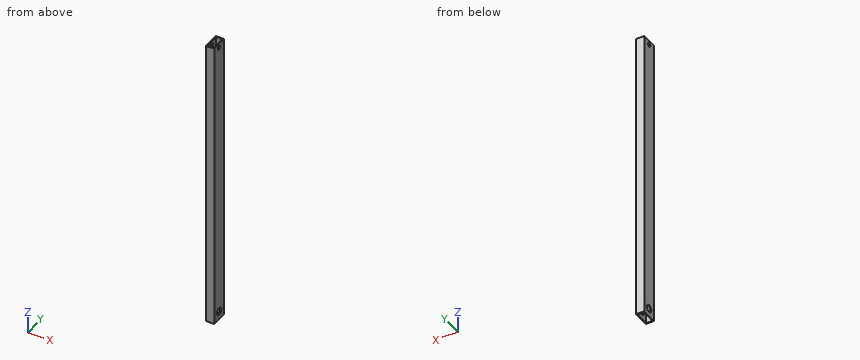
Autodesk Inventor part; units mm, degrees
ref_plane "YZ Plane" through (0, 0, 0) normal (1, 0, 0) x (0, 1, 0)
ref_plane "XZ Plane" through (0, 0, 0) normal (0, 1, 0) x (-1, 0, 0)
ref_plane "XY Plane" through (0, 0, 0) normal (0, 0, 1) x (1, 0, 0)
sketch "Sketch1" plane through (0, 0, 0) normal (0, 0, 1) x (1, 0, 0)
  line L0 (0, 0) -> (25.4, 0)
  line L1 (25.4, 0) -> (25.4, 50.8)
  line L2 (25.4, 50.8) -> (0, 50.8)
  line L3 (0, 50.8) -> (0, 0)
  dimension "d0" = 25.4
  dimension "d1" = 50.8
extrude "Extrusion1" add sketch "Sketch1" along normal blind 914.4
shell "Shell1" thickness 3.175 removed faces 2 at (8.4667, 16.9333, 0) at (8.4667, 16.9333, 914.4)
sketch "Sketch2" plane through (25.4, 0, 0) normal (1, 0, 0) x (0, 0, -1)
  circle A0 centre (-25.4, 25.4) radius 11.43
  line L0 (0, 50.8) -> (-914.4, 50.8)
  line L1 (0, 0) -> (0, 50.8)
  circle A1 centre (-901.7, 25.4) radius 6.35
  line L2 (-914.4, 0) -> (-914.4, 50.8)
  dimension "d5" = 22.86
  dimension "d6" = 25.4
  dimension "d7" = 25.4
  dimension "d10" = 12.7
  dimension "d11" = 25.4
  dimension "d12" = 12.7
extrude "Extrusion2" cut sketch "Sketch2" against normal blind 25.4
properties part number "Kermit Frame 17"
Check sheet for the modelled part. Datum: model origin and axes. Units: mm. Round coordinates to 2 decimals unless told otherwise and drop trailing zeros. Loops run counter-clockwise (first coordinate to the right, second up) from the corner with the lowest first, then second, coordinate; pieces in that order, holes last. Notation, with made-up numbers: (-3, -33) -> (29, -33) arc R17 ccw to (29, 0) -> close; hole circle Ø7 at (27, 74.25). An arc over 180 degrees is marked (long way). Write item = value, one per line. Start each with the question number.
1) Sectioned sample at A-A, the plane z = 25.4. Record the cut outline in (x, y) (3 decimals), plus the area to 3 significant figures.
2) Sectioned sample at B-B, the plane z = 830. Record the cut outline in (x, y) (3 decimals), plus the area to 3 significant figures.
3) Thickness scan on probe 1 along X at (y, z) = (15, 677) (3 decimals); probe 2 along Y at (x, z) = (5.5, 214.5) (3 decimals); probe 3 along Y at (x, z) = (2.1, 901.7). Record the ranges inside material, lowest first.
Results are:
q1.outline = (0, 0) -> (25.4, 0) -> (25.4, 13.97) -> (22.225, 13.97) -> (22.225, 3.175) -> (3.175, 3.175) -> (3.175, 13.97) -> (0, 13.97) -> close; (0, 36.83) -> (3.175, 36.83) -> (3.175, 47.625) -> (22.225, 47.625) -> (22.225, 36.83) -> (25.4, 36.83) -> (25.4, 50.8) -> (0, 50.8) -> close
q1.area = 298 mm^2
q2.outline = (0, 0) -> (25.4, 0) -> (25.4, 50.8) -> (0, 50.8) -> close; hole (3.175, 3.175) -> (22.225, 3.175) -> (22.225, 47.625) -> (3.175, 47.625) -> close
q2.area = 444 mm^2
q3.probe_1 = 0 to 3.175, 22.225 to 25.4
q3.probe_2 = 0 to 3.175, 47.625 to 50.8
q3.probe_3 = 0 to 19.05, 31.75 to 50.8
